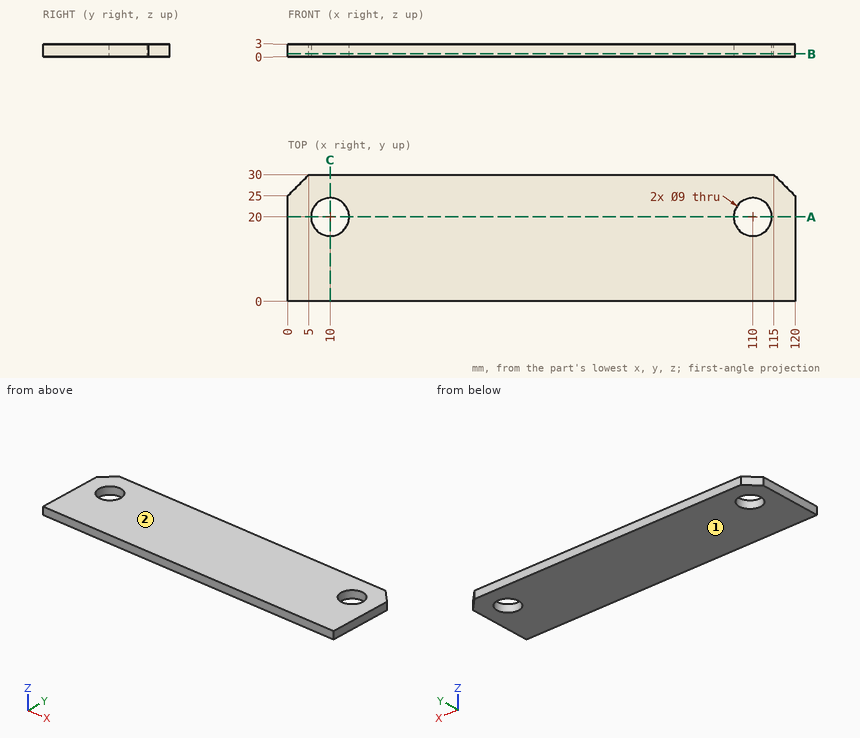
Geometry: see drawing. Coordinates: mm, zero at the bounding-box minimum. Round coordinates to 2 decimals unless told otherwise and drop trailing zeros. Write each loop counter-clockwise with the first axis right and the second up, starting at its lowest first coordinate (ties: lowest second). Pieces come first, ordered by that corner, then holes.
Item 1: Mould query, pull axis Z, two halves, no side actions, for the marked faces 1 and 2. Classes: +Z half, -Z half, draft (parallel to the pull), parting line (faces both ways), or undercut.
Item 2: Section query A-A (y = 20). Return loops of the section in (x, z).
Item 3: Section query C-C (x = 10). Return loops of the section in (y, z), plus the area to 3 significant figures.
Item 4: Pin query (flat end, axial travel): P1, Ø1, axis at x = 77, z = 0.5, coming from the -Y side. Return the tip coordinate at first contact, or that it passes through.
Item 5: Material intervals for L1, parallel to Y at x = 10, z = 1.7; L2, parallel to X at y = 18.5, z = 0.5; L3, parallel to Y at x = 112, z = 1.4, sorted ascending.
Item 6: Section query B-B (z = 0.65). Return loops of the section in (x, y).
Completed:
1. face 1: -Z half
1. face 2: +Z half
2. outline: (0, 0) - (5.5, 0) - (5.5, 3) - (0, 3) - close; (14.5, 0) - (105.5, 0) - (105.5, 3) - (14.5, 3) - close; (114.5, 0) - (120, 0) - (120, 3) - (114.5, 3) - close
3. outline: (0, 0) - (15.5, 0) - (15.5, 3) - (0, 3) - close; (24.5, 0) - (30, 0) - (30, 3) - (24.5, 3) - close
3. area: 63.0 mm2
4. P1: stops at y = 0
5. L1: y = 0 to 15.5, 24.5 to 30
5. L2: x = 0 to 5.76, 14.24 to 105.76, 114.24 to 120
5. L3: y = 0 to 15.97, 24.03 to 30
6. outline: (0, 0) - (120, 0) - (120, 25) - (115, 30) - (5, 30) - (0, 25) - close; hole circle Ø9 at (10, 20); hole circle Ø9 at (110, 20)
